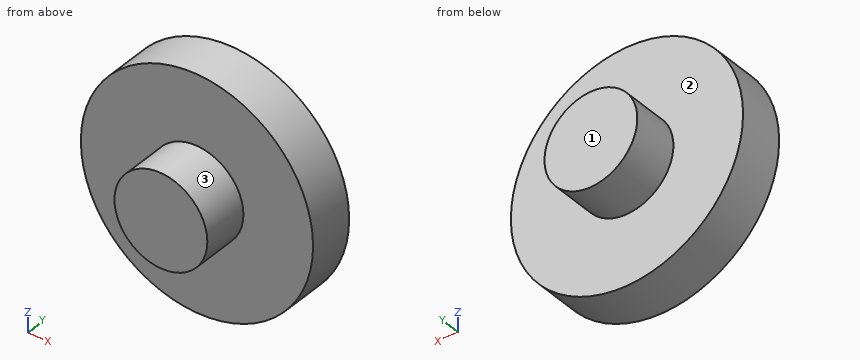
from build123d import *

# Parameters (mm, degrees)
F0_R     = 10
F1_DEPTH = 15
F2_DEPTH = 15
F0_R_2   = 25
F3_DEPTH = 5
F4_DEPTH = 5


with BuildPart() as f1:
    # F0 (on Front) → F1 (new body)
    with BuildSketch(Plane.XZ):
        Circle(F0_R)
    extrude(amount=F1_DEPTH)

    # F0 (on Front) → F2 (join)
    with BuildSketch(Plane.XZ):
        Circle(F0_R)
    extrude(amount=-F2_DEPTH)

    # F0 (on Front) → F3 (join)
    with BuildSketch(Plane.XZ):
        Circle(F0_R_2)
        Circle(F0_R, mode=Mode.SUBTRACT)
    extrude(amount=F3_DEPTH)

    # F0 (on Front) → F4 (join)
    with BuildSketch(Plane.XZ):
        Circle(F0_R_2)
        Circle(F0_R, mode=Mode.SUBTRACT)
    extrude(amount=-F4_DEPTH)


solid = f1.part
Part model, mm, in its own coordinate system. Face numbers are marked on the shaded views. A direction names the side the tool comes from. Coordinates: 2 decimals unless noted, no trailing zeros. Order: outer loops, then holes, each group sorted by start corner. A loop starts at its lowest first (then second) coordinate and runs counter-clockwise, first axis right, second up.
(1) Slice it at D-D, the plane y = 8. Write the cut outline in (x, z), and give its area (3 significant figures).
Check sheet entries:
outline: circle Ø20 at (0, 0)
area: 314 mm2
(2) Slice it at B-B, the plane x = 0. Write the cut outline in (y, z).
Check sheet entries:
outline: (-15, -10) - (-5, -10) - (-5, -25) - (5, -25) - (5, -10) - (15, -10) - (15, 10) - (5, 10) - (5, 25) - (-5, 25) - (-5, 10) - (-15, 10) - close
(3) Pin check, flat tips, straight feed: pin 1 Ø6 at (x, y) = (-14, 11) entering from -Z; pin 2 Ø12 at (x, y) = (-18.5, 0.5) entering from +Z; pin 3 Ø4 at (x, y) = (13, 0.5) entering from -Z; pin 4 Ø4 at (x, z) = (14.5, 14) entering from -Y. Stop position of each tip, or through.
Check sheet entries:
pin 1: passes through
pin 2: stops at z = 21.65
pin 3: stops at z = -22.45
pin 4: stops at y = -5
(4) Tool access for the marked faces 1, 2 and 3: list every direction of +Z, -Z, +X, -X, +Y, -Y with a clear straight run to the whole face (end or side of a thin tool).
Check sheet entries:
face 1: +Z, -Z, +X, -X, +Y
face 2: +Y
face 3: -Y
(5) Probe L1, parallel to Y at x = 11, z = 17; L2, parallel to Z at x = 0.5, y = 6; L3, parallel to X at y = 1.5, z = -6. List the from-to ranges inside material, lowest first.
Check sheet entries:
L1: y = -5 to 5
L2: z = -9.99 to 9.99
L3: x = -24.27 to 24.27
(6) Slice it at C-C, the plane y = -3.75. Write the cut outline in (x, z), and give its area (3 significant figures).
Check sheet entries:
outline: circle Ø50 at (0, 0)
area: 1,960 mm2
(7) Slice it at A-A, the plane z = 0. Write the cut outline in (x, y).
Check sheet entries:
outline: (-25, -5) - (-10, -5) - (-10, -15) - (10, -15) - (10, -5) - (25, -5) - (25, 5) - (10, 5) - (10, 15) - (-10, 15) - (-10, 5) - (-25, 5) - close
